```python
from build123d import *

# Parameters (mm, degrees)
SKETCH_W        = 32.240891
SKETCH_H        = 17.088121
PAD_DEPTH       = 2.6
SKETCH002_R     = 1.28
SKETCH002_W     = 22.850001
SKETCH002_H     = 11.84
POCKET_DEPTH    = 2.6
SKETCH003_W     = 2.01
SKETCH003_H     = 3.5
POCKET001_DEPTH = 5


with BuildPart() as part:
    # Sketch → Pad (new body)
    with BuildSketch(Plane.XZ):
        with Locations((16.120445, 8.54406)):
            Rectangle(SKETCH_W, SKETCH_H)
    extrude(amount=PAD_DEPTH)

    # Sketch002 (on Face6 of Pad) → Pocket (cut)
    with BuildSketch(Plane.XZ.offset(2.6)):
        with Locations((30.105934, 8.54406)):
            Circle(SKETCH002_R)
        with Locations((2.134957, 8.54406)):
            Circle(SKETCH002_R)
        with Locations((16.120445, 8.544061)):
            Rectangle(SKETCH002_W, SKETCH002_H)
    extrude(amount=-POCKET_DEPTH, mode=Mode.SUBTRACT)

    # Sketch003 (on Face4 of Pocket) → Pocket001 (cut)
    with BuildSketch(Plane(origin=(0, 0, 0), x_dir=(1, 0, 0), z_dir=(0, 1, 0))):
        with Locations((27.953742, -8.544061)):
            Rectangle(SKETCH003_W, SKETCH003_H)
    extrude(amount=-POCKET001_DEPTH, mode=Mode.SUBTRACT)


solid = part.part
```
Geometry check sheet. Reference: the model listing, model coordinates, mm. A direction names the side the tool comes from. Round coordinates to 2 decimals unless told otherwise and drop trailing zeros. Loops run counter-clockwise (first coordinate to the right, second up) from the corner with the lowest first, then second, coordinate; pieces in that order, holes last. Notation, with made-up numbers: (-16.5, 12) - (-11.5, 12) arc R11 ccw to (-11.5, 20) - close; hole circle Ø6 at (2.25, -26.75). An arc over 180 degrees is marked (long way). Write each question's results on one line, items separated by ' | '. Start each with the question number.
Q1. Cross-section at A-A on x = 18. Enter the section's corners in (y, z), and give its area (3 significant figures).
Q2. Thickness scan on line 1 (Z direction, x = 5, y = -0.55); line 2 (X direction, y = -1.6, z = 13); line 3 (Z direction, x = 28, y = -0.3). Record the ranges inside material, lowest first. Write a range as [from, to].
Q3. Release check for a two-part mould opening along X. For faces 3 (the flat face through (0, -1, 8)), 4 (the flat face through (16, -1, 17.088)), 5 (the cylindrical face through (31.385, -1.318, 8.496)), 6 (the flat face through (16, -1, 14.464)) record: +X half, -X half, draft (parallel to the pull), parting line (faces both ways), or undercut.
Q4. Access from +Z, -Z, +X, -X, +Y, -Y to the whole of each face (thin tool, end or side, straight path). Record for faces 1 (the flat face through (16, 0, 16)), 2 (the flat face through (27.545, -1, 5)).
Q5. Cross-section at D-D on z = 9.5. Enter the section's corners in (x, y).
Q6. Cross-section at C-C on y = -2.3. Enter the section's corners in (x, z).
Q7. Gauge pin test, flat end, axial feed: P1, Ø4, axis at x = 17.5, z = 11.5, coming from the +Y side. Record the tip position at first contact, or that the pin passes through.
Q8. Cross-section at B-B on z = 12. Enter the section's corners in (x, y), and give its area (3 significant figures).
Answers below:
1) outline: (-2.6, 0) - (0, 0) - (0, 2.62) - (-2.6, 2.62) - close; (-2.6, 14.46) - (0, 14.46) - (0, 17.09) - (-2.6, 17.09) - close | area: 13.6 mm²
2) line 1: z = [0, 2.62], [14.46, 17.09] | line 2: x = [0, 4.7], [27.55, 32.24] | line 3: z = [0, 6.79], [10.29, 17.09]
3) face 3: -X half | face 4: draft | face 5: undercut | face 6: undercut
4) face 1: +Z, -Z, +X, -X, +Y | face 2: +Y, -Y
5) outline: (0, -2.6) - (1.28, -2.6) - (1.28, 0) - (0, 0) - close; (2.99, -2.6) - (4.7, -2.6) - (4.7, 0) - (2.99, 0) - close; (28.96, -2.6) - (29.25, -2.6) - (29.25, 0) - (28.96, 0) - close; (30.96, -2.6) - (32.24, -2.6) - (32.24, 0) - (30.96, 0) - close
6) outline: (0, 0) - (32.24, 0) - (32.24, 17.09) - (0, 17.09) - close; hole circle Ø2.56 at (2.13, 8.54); hole (4.7, 2.62) - (27.55, 2.62) - (27.55, 6.79) - (28.96, 6.79) - (28.96, 7.98) arc R1.28 ccw (long way) to (28.96, 9.11) - (28.96, 10.29) - (27.55, 10.29) - (27.55, 14.46) - (4.7, 14.46) - close
7) P1: passes through
8) outline: (0, -2.6) - (4.7, -2.6) - (4.7, 0) - (0, 0) - close; (27.55, -2.6) - (32.24, -2.6) - (32.24, 0) - (27.55, 0) - close | area: 24.4 mm²
